```python
from build123d import *

# Parameters (mm, degrees)
F1_DEPTH = 25
F2_DEPTH = 10
F0_W     = 20
F0_H     = 30
F3_DEPTH = 15


with BuildPart() as f1:
    # F0 (on Top) → F1 (new body)
    with BuildSketch(Plane.XY):
        Polygon((0, 25), (0, 0), (5, 0), (25, 0), (25, 25), align=None)
    extrude(amount=F1_DEPTH)

    # F0 (on Top) → F2 (join)
    with BuildSketch(Plane.XY):
        Polygon((5, 0), (0, 0), (0, 25), (-25, 25), (-25, -30), (5, -30), align=None)
    extrude(amount=F2_DEPTH)

    # F0 (on Top) → F3 (join)
    with BuildSketch(Plane.XY):
        with Locations((15, -15)):
            Rectangle(F0_W, F0_H)
    extrude(amount=F3_DEPTH)


solid = f1.part
```
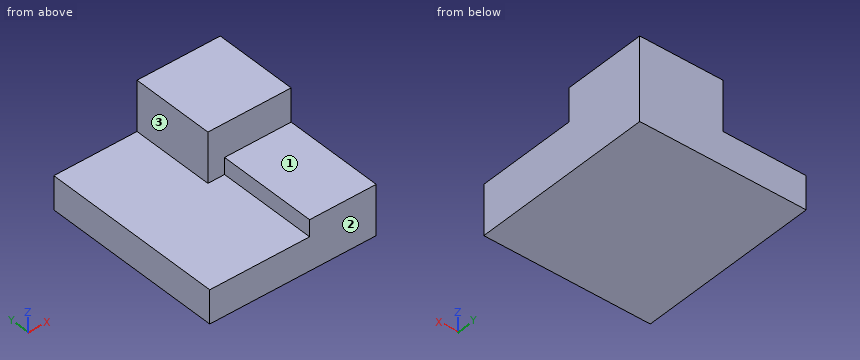
Geometry: final body of the model. Coordinates: model frame, mm. Face numbers are marked on the shaded views. A direction names the side the tool comes from. Coordinates: 2 decimals unless noted, no trailing zeros. Loops run counter-clockwise (first coordinate to the right, second up) from the corner with the lowest first, then second, coordinate; pieces in that order, holes last. Notation, with made-up numbers: M 23.5,83.25 L 34.5,83.25 A23 cw 34.5,99.25 Z; hole C -26,4 d1. An arc over 180 degrees is marked long. Put each result on its own line as item: value.
(1) Cut plane B-B on y = 9. Return the cut outline in (x, z).
Answer sheet:
outline: M -25,0 L 25,0 L 25,25 L 0,25 L 0,10 L -25,10 Z
(2) First-contact query: pin 1 (6 mm diameter, centred on y = -3.5, z = 21.5, fed in from +X); pin 2 (8 mm diameter, centred on y = 7, z = 15.5, fed in from -X); pin 3 (6 mm diameter, centred on x = 13.5, y = -16.5, fed in from +Z); pin 4 (5.5 mm diameter, centred on y = -20.5, z = 13, fed in from -X). Flat tips, straight axial feed; report the tip coordinate or a pass-through.
Answer sheet:
pin 1: passes through
pin 2: stops at x = 0
pin 3: stops at z = 15
pin 4: stops at x = 5
(3) Access query for the marked faces 1, 2 and 3. Directions: +Z, -Z, +X, -X, +Y, -Y. A direction counts if a zero-diameter tool reaches every point of the face in a straight line with its end or side. Return the directions, or none.
Answer sheet:
face 1: +Z, +X, -X, -Y
face 2: +Z, -Z, +X, -X, -Y
face 3: +Z, -X, +Y, -Y
(4) Cut plane C-C on x = -17. Return the cut outline in (y, z), then the cut area to 3 significant figures.
Answer sheet:
outline: M -30,0 L 25,0 L 25,10 L -30,10 Z
area: 550 mm^2
(5) Material intervals for probe 1 along Z at (x, y) = (14, -14.5); probe 2 along Z at (x, y) = (-19, 2.5); probe 3 along Y at (x, z) = (20.5, 23.25), sorted ascending.
Answer sheet:
probe 1: z = 0 to 15
probe 2: z = 0 to 10
probe 3: y = 0 to 25
(6) Cut plane A-A on x = 1. Return the cut outline in (y, z), then the cut area to 3 significant figures.
Answer sheet:
outline: M -30,0 L 25,0 L 25,25 L 0,25 L 0,10 L -30,10 Z
area: 925 mm^2
